Verification items for this drawing (mm, ordinates from the low corner). Round coordinates to 2 decimals unless told otherwise and drop trailing zeros. Write each loop counter-clockwise with the first axis right and the second up, starting at its lowest first coordinate (ties: lowest second). Pieces come first, ordered by that corner, then holes. Notation, with made-up numbers: (-35, -16.5) -> (23, -16.5) arc R28 cw to (23, 7.5) -> close; hole circle Ø11 at (78.25, -2.5). An arc over 180 degrees is marked (long way). Use one line per item in the form item = value. Start each with the question number.
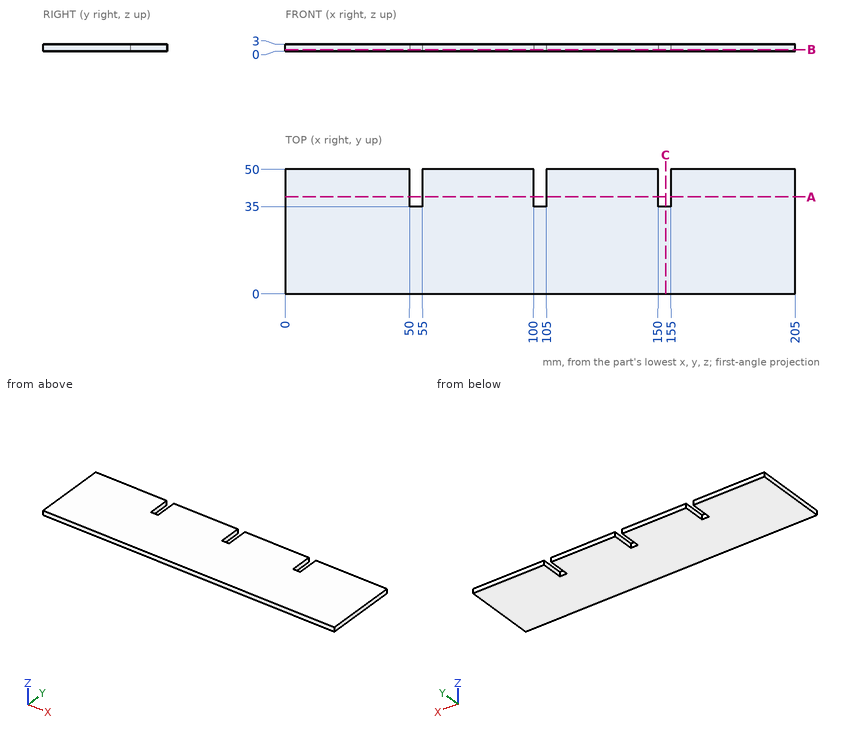
1. Sectioned sample at A-A (y = 39). Enter the section's corners in (x, z), and give its area (3 significant figures).
2. Sectioned sample at B-B (z = 0.75). Enter the section's corners in (x, y).
3. Sectioned sample at C-C (x = 153). Enter the section's corners in (y, z), and give its area (3 significant figures).
4. Depth check by flat-ended pin: pin 1 (1.5 mm diameter, centred on x = 151.5, z = 1, fed in from +Y). Enter the tip coordinate at first touch or a pass-through.
5. Scan line: probe 1 along X at (y, z) = (45, 1.25). Record every from-to range of solid material in increasing order.
Returned:
q1.outline = (0, 0) -> (50, 0) -> (50, 3) -> (0, 3) -> close; (55, 0) -> (100, 0) -> (100, 3) -> (55, 3) -> close; (105, 0) -> (150, 0) -> (150, 3) -> (105, 3) -> close; (155, 0) -> (205, 0) -> (205, 3) -> (155, 3) -> close
q1.area = 570 mm^2
q2.outline = (0, 0) -> (205, 0) -> (205, 50) -> (155, 50) -> (155, 35) -> (150, 35) -> (150, 50) -> (105, 50) -> (105, 35) -> (100, 35) -> (100, 50) -> (55, 50) -> (55, 35) -> (50, 35) -> (50, 50) -> (0, 50) -> close
q3.outline = (0, 0) -> (35, 0) -> (35, 3) -> (0, 3) -> close
q3.area = 105 mm^2
q4.pin_1 = 35
q5.probe_1 = 0 to 50, 55 to 100, 105 to 150, 155 to 205
